Input: part model. Units: mm. Frame: model coordinates. Face numbers are marked on the shaded views. A direction names the side the tool comes from. Round coordinates to 2 decimals unless told otherwise and drop trailing zeros. Order: outer loops, then holes, each group sorted by start corner. A loop starts at its lowest first (then second) coordinate and runs counter-clockwise, first axis right, second up. Notation, with made-up numbers: (-10.75, -25) - (7.25, -25) arc R9 ccw to (7.25, -20) - close; hole circle Ø8 at (-31.5, 82.5). An arc over 180 degrees is marked (long way). One line per item, written item: value. Start each with the question number.
Autodesk Inventor part; units mm, degrees
ref_plane "YZ Plane" through (0, 0, 0) normal (1, 0, 0) x (0, 1, 0)
ref_plane "XZ Plane" through (0, 0, 0) normal (0, 1, 0) x (-1, 0, 0)
ref_plane "XY Plane" through (0, 0, 0) normal (0, 0, 1) x (1, 0, 0)
sketch "Sketch1" plane through (0, 0, 0) normal (0, 0, 1) x (1, 0, 0)
  line L0 (-34.86, 0) -> (34.86, 0) construction
  line L1 (0, -34.86) -> (0, 34.86) construction
  line L2 (0, 0) -> (11.1575, 11.1575) construction
  line L3 (0, 0) -> (15.7791, 0) construction
  line L4 (0, 24.9) -> (16.8009, 24.9)
  line L5 (16.8009, 24.9) -> (16.8009, 21.2415)
  line L6 (16.8009, 21.2415) -> (19.0212, 19.0212)
  line L7 (24.9, 0) -> (24.9, 16.8009)
  line L8 (24.9, 16.8009) -> (21.2415, 16.8009)
  line L9 (21.2415, 16.8009) -> (19.0212, 19.0212)
  line L10 (0, -24.9) -> (16.8009, -24.9)
  line L11 (16.8009, -24.9) -> (16.8009, -21.2415)
  line L12 (16.8009, -21.2415) -> (19.0212, -19.0212)
  line L13 (24.9, 0) -> (24.9, -16.8009)
  line L14 (24.9, -16.8009) -> (21.2415, -16.8009)
  line L15 (21.2415, -16.8009) -> (19.0212, -19.0212)
  line L16 (0, 24.9) -> (-16.8009, 24.9)
  line L17 (-16.8009, 24.9) -> (-16.8009, 21.2415)
  line L18 (-16.8009, 21.2415) -> (-19.0212, 19.0212)
  line L19 (-24.9, 16.8009) -> (-21.2415, 16.8009)
  line L20 (-21.2415, 16.8009) -> (-19.0212, 19.0212)
  line L21 (0, -24.9) -> (-16.8009, -24.9)
  line L22 (-16.8009, -24.9) -> (-16.8009, -21.2415)
  line L23 (-16.8009, -21.2415) -> (-19.0212, -19.0212)
  line L24 (-21.2415, -16.8009) -> (-19.0212, -19.0212)
  line L25 (-24.9, -16.8009) -> (-21.2415, -16.8009)
  line L26 (-24.9, 0) -> (-24.9, -16.8009)
  line L27 (-24.9, 0) -> (-24.9, 16.8009)
  circle A0 centre (0, 0) radius 12.5
  dimension "d0" = 45
  dimension "d2" = 24.9
  dimension "d3" = 3.14
  dimension "d4" = 26.9
  dimension "d5" = 25
extrude "Extrusion1" add sketch "Sketch1" along normal blind 5
sketch "Sketch2" plane through (0, 0, 5) normal (0, 0, 1) x (1, 0, 0)
  circle A0 centre (0, 0) radius 12.5
  line L0 (16.8009, 24.9) -> (-16.8009, 24.9)
  line L1 (-16.8009, 24.9) -> (-16.8009, 21.2415)
  line L2 (-16.8009, 21.2415) -> (-21.2415, 16.8009)
  line L3 (-21.2415, 16.8009) -> (-24.9, 16.8009)
  line L4 (-24.9, 16.8009) -> (-24.9, -16.8009)
  line L5 (-24.9, -16.8009) -> (-21.2415, -16.8009)
  line L6 (-21.2415, -16.8009) -> (-16.8009, -21.2415)
  line L7 (-16.8009, -21.2415) -> (-16.8009, -24.9)
  line L8 (-16.8009, -24.9) -> (16.8009, -24.9)
  line L9 (16.8009, -24.9) -> (16.8009, -21.2415)
  line L10 (16.8009, -21.2415) -> (21.2415, -16.8009)
  line L11 (21.2415, -16.8009) -> (24.9, -16.8009)
  line L12 (24.9, -16.8009) -> (24.9, 16.8009)
  line L13 (24.9, 16.8009) -> (21.2415, 16.8009)
  line L14 (21.2415, 16.8009) -> (16.8009, 21.2415)
  line L15 (16.8009, 21.2415) -> (16.8009, 24.9)
  line L16 (-34.86, 0) -> (34.86, 0) construction
  line L17 (0, -34.86) -> (0, 34.86) construction
  line L18 (-10, 21.9) -> (10, 21.9)
  line L19 (10, 21.9) -> (10, 18.9)
  line L20 (10, 18.9) -> (-10, 18.9)
  line L21 (-10, 18.9) -> (-10, 21.9)
  line L22 (-10, -21.9) -> (10, -21.9)
  line L23 (10, -21.9) -> (10, -18.9)
  line L24 (10, -18.9) -> (-10, -18.9)
  line L25 (-10, -18.9) -> (-10, -21.9)
  dimension "d8" = 20
  dimension "d9" = 3
  dimension "d10" = 3
extrude "Extrusion2" add sketch "Sketch2" along normal blind 7 contours L18 L19 L20 L21 | L25 L24 L23 L22
chamfer "Fase1" [suppressed]
chamfer "Fase2" [suppressed]
sketch "Sketch4" plane through (0, 0, 0) normal (0, 0, -1) x (-1, 0, 0)
  circle A0 centre (0, 0) radius 12.5 construction
  line L0 (16.8009, 24.9) -> (-16.8009, 24.9) construction
  line L1 (-16.8009, 24.9) -> (-16.8009, 21.2415)
  line L2 (-16.8009, 21.2415) -> (-21.2415, 16.8009)
  line L3 (-21.2415, 16.8009) -> (-24.9, 16.8009)
  line L4 (-24.9, 16.8009) -> (-24.9, -16.8009) construction
  line L5 (-24.9, -16.8009) -> (-21.2415, -16.8009)
  line L6 (-21.2415, -16.8009) -> (-16.8009, -21.2415)
  line L7 (-16.8009, -21.2415) -> (-16.8009, -24.9)
  line L8 (-16.8009, -24.9) -> (16.8009, -24.9) construction
  line L9 (16.8009, -24.9) -> (16.8009, -21.2415)
  line L10 (16.8009, -21.2415) -> (21.2415, -16.8009)
  line L11 (21.2415, -16.8009) -> (24.9, -16.8009)
  line L12 (24.9, -16.8009) -> (24.9, 16.8009) construction
  line L13 (24.9, 16.8009) -> (21.2415, 16.8009)
  line L14 (21.2415, 16.8009) -> (16.8009, 21.2415)
  line L15 (16.8009, 21.2415) -> (16.8009, 24.9)
  line L16 (-17.0009, 25.1) -> (17.0009, 25.1) construction
  line L17 (17.0009, 25.1) -> (17.0009, 21.3243)
  line L18 (17.0009, 21.3243) -> (21.3243, 17.0009)
  line L19 (21.3243, 17.0009) -> (25.1, 17.0009)
  line L20 (25.1, 17.0009) -> (25.1, -17.0009) construction
  line L21 (25.1, -17.0009) -> (21.3243, -17.0009)
  line L22 (21.3243, -17.0009) -> (17.0009, -21.3243)
  line L23 (17.0009, -21.3243) -> (17.0009, -25.1)
  line L24 (17.0009, -25.1) -> (-17.0009, -25.1) construction
  line L25 (-17.0009, -25.1) -> (-17.0009, -21.3243)
  line L26 (-17.0009, -21.3243) -> (-21.3243, -17.0009)
  line L27 (-21.3243, -17.0009) -> (-25.1, -17.0009)
  line L28 (-25.1, -17.0009) -> (-25.1, 17.0009) construction
  line L29 (-25.1, 17.0009) -> (-21.3243, 17.0009)
  line L30 (-21.3243, 17.0009) -> (-17.0009, 21.3243)
  line L31 (-17.0009, 21.3243) -> (-17.0009, 25.1)
  line L32 (-24.9, -16.8009) -> (-24.9, 16.8009)
  line L33 (-24.9, 16.8009) -> (-24.9, 17.0009)
  line L34 (-16.8009, 24.9) -> (-17.0009, 24.9)
  line L35 (-16.8009, 24.9) -> (16.8009, 24.9)
  line L36 (16.8009, 24.9) -> (17.0009, 24.9)
  line L37 (24.9, 16.8009) -> (24.9, 17.0009)
  line L38 (24.9, 16.8009) -> (24.9, -16.8009)
  line L39 (24.9, -16.8009) -> (24.9, -17.0009)
  line L40 (16.8009, -24.9) -> (-16.8009, -24.9)
  line L41 (16.8009, -24.9) -> (17.0009, -24.9)
  line L42 (-16.8009, -24.9) -> (-17.0009, -24.9)
  line L43 (-24.9, -16.8009) -> (-24.9, -17.0009)
  dimension "d19" = 0.2
extrude "IM_offset" add sketch "Sketch4" against normal up to surface (5 mm away) contours L1 L2 L3 L33 L29 L30 L31 L34 | L36 L17 L18 L19 L37 L13 L14 L15 | L5 L6 L7 L42 L25 L26 L27 L43 | L39 L21 L22 L23 L41 L9 L10 L11
properties part number "20_Cube_insert_Sample_holder_v3"
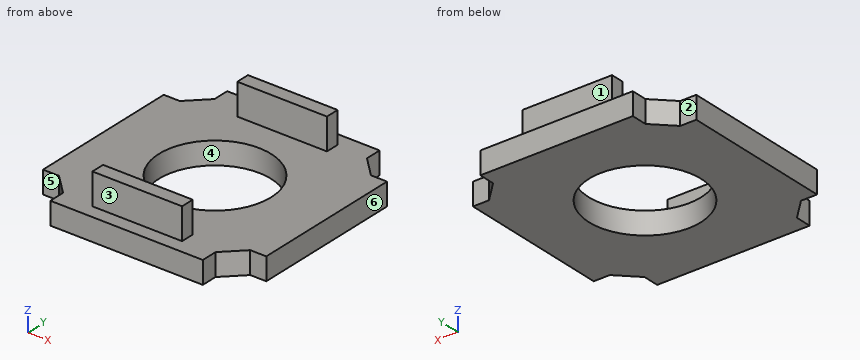
Item 1: Section query A-A on x = 0. Return loops of the section in (y, z).
Item 2: Pull-direction query (X, two-part tool) for the marked faces 4, 5 and 6; classes: released by +X, released by -X, zero draft, split by the parting line, or undercut.
Item 3: Section query C-C on y = 0. Return loops of the section in (x, z).
Item 4: Section query D-D on z = 1.5. Return loops of the section in (x, y), and give its area (3 significant figures).
Item 5: Section query B-B on z = 8. Return loops of the section in (x, y), and give its area (3 significant figures).
Item 6: Reachability of the marked faces 1, 2 and 3 from +Z, -Z, +X, -X, +Y, -Y: full face, straight path, thin tool, end or side. Return the list, or none.
Item 7: First-contact query: pin 1 Ø1.8 at (y, z) = (-22.5, 3.5) entering from -X; pin 2 Ø15 at (x, y) = (12.5, 2) entering from +Z; pin 3 Ø2 at (x, z) = (-4, 10) entering from +Y; pin 4 Ø5 at (y, z) = (-3, 9.5) entering from +X. Flat tips, straight axial feed; report the tip coordinate or a pass-through.
Item 8: Line query: L1, parallel to Y at x = -1.5, z = 11; L2, parallel to Y at x = 0, z = 2.8; L3, parallel to Z at x = 22, y = -15.5. Output: solid intervals per line, ascending.
Geometry results:
1. outline: (-24.9, 0) - (-12.5, 0) - (-12.5, 5) - (-18.9, 5) - (-18.9, 12) - (-21.9, 12) - (-21.9, 5) - (-24.9, 5) - close; (12.5, 0) - (24.9, 0) - (24.9, 5) - (21.9, 5) - (21.9, 12) - (18.9, 12) - (18.9, 5) - (12.5, 5) - close
2. face 4: undercut
2. face 5: zero draft
2. face 6: released by +X
3. outline: (-24.9, 0) - (-12.5, 0) - (-12.5, 5) - (-24.9, 5) - close; (12.5, 0) - (24.9, 0) - (24.9, 5) - (12.5, 5) - close
4. outline: (-24.9, -17) - (-21.32, -17) - (-17, -21.32) - (-17, -24.9) - (17, -24.9) - (17, -21.32) - (21.32, -17) - (24.9, -17) - (24.9, 17) - (21.32, 17) - (17, 21.32) - (17, 24.9) - (-17, 24.9) - (-17, 21.32) - (-21.32, 17) - (-24.9, 17) - close; hole circle Ø25 at (0, 0)
4. area: 1,780 mm^2
5. outline: (-10, -21.9) - (10, -21.9) - (10, -18.9) - (-10, -18.9) - close; (-10, 18.9) - (10, 18.9) - (10, 21.9) - (-10, 21.9) - close
5. area: 120 mm^2
6. face 1: +Z, +X, -X, +Y
6. face 2: +Z, -Z, -X, +Y
6. face 3: +Z, +X, -X, -Y
7. pin 1: stops at x = -17
7. pin 2: stops at z = 5
7. pin 3: stops at y = 21.9
7. pin 4: passes through
8. L1: y = -21.9 to -18.9, 18.9 to 21.9
8. L2: y = -24.9 to -12.5, 12.5 to 24.9
8. L3: z = 0 to 5
